Autodesk Inventor part; units mm, degrees
ref_plane "C3_XY" through (39.5, 0, 0) normal (-1, 0, 0) x (0, 0, -1)
ref_plane "C3_YZ" through (39.5, 0, 0) normal (0, 0, -1) x (0, -1, 0)
ref_plane "C3_ZX" through (39.5, 0, 0) normal (0, -1, 0) x (-1, 0, 0)
sketch "Sketch_1" plane through (0, 0, 0) normal (0, 0, 1) x (1, 0, 0)
  line L0 (39.5, 0) -> (0, 0)
  line L1 (0, 0) -> (0, 3)
  line L2 (0, 3) -> (0.5485, 3.95)
  line L3 (0.5485, 3.95) -> (38.9515, 3.95)
  line L4 (38.9515, 3.95) -> (39.5, 3)
  line L5 (39.5, 3) -> (39.5, 0)
  line L6 (39.5, 0) -> (0, 0)
revolve "Revolution1" add sketch "Sketch_1" angle 360 about axis through (39.5, 0, 0) along (1, 0, 0)
sketch "Sketch_2" plane through (0, 0, 0) normal (1, 0, 0) x (0, 1, 0)
  line L0 (6, 6) -> (-6, 6)
  line L1 (-6, 6) -> (-6, -6)
  line L2 (-6, -6) -> (6, -6)
  line L3 (6, -6) -> (6, 6)
  line L4 (-1.7321, 3) -> (-3.4641, 0)
  line L5 (-3.4641, 0) -> (-1.7321, -3)
  line L6 (-1.7321, -3) -> (1.7321, -3)
  line L7 (1.7321, -3) -> (3.4641, 0)
  line L8 (3.4641, 0) -> (1.7321, 3)
  line L9 (1.7321, 3) -> (-1.7321, 3)
extrude "Extrusion1" cut sketch "Sketch_2" along normal blind 39.5
sketch "Sketch3" plane through (0, 0, 0) normal (-1, 0, 0) x (0, 0, 1)
  point P0 (0, 0)
hole "Hole1" at (0, 0, 0) direction (1, 0, 0) diameter 2.459 depth 8.2901 tip angle 120 countersink diameter 3 countersink angle 90
sketch "Sketch4" plane through (39.5, 0, 0) normal (1, 0, 0) x (0, 0, -1)
  point P0 (0, 0)
hole "Hole2" at (39.5, 0, 0) direction (-1, 0, 0) diameter 2.459 depth 8.2901 tip angle 120 countersink diameter 3 countersink angle 90
ref_plane "C3_XY" through (39.5, 0, 0) normal (-1, 0, 0) x (0, 0, -1)
ref_plane "C3_YZ" through (39.5, 0, 0) normal (0, 0, -1) x (0, -1, 0)
ref_plane "C3_ZX" through (39.5, 0, 0) normal (0, -1, 0) x (-1, 0, 0)
properties part number "SLSBF6-39.5-M3-N3"
Input: part model. Units: mm. Frame: model coordinates. A direction names the side the tool comes from. Give positions to 0.01 mm unless a question says otherwise; leave off trailing zeros. Order: outer loops, then holes, each group sorted by start corner. A loop starts at its lowest first (then second) coordinate and runs counter-clockwise, first axis right, second up. Notation, with made-up numbers: M -35,28.5 L -11,28.5 A35 ccw -11,62.5 Z; hole C 21,55.5 d1. An arc over 180 degrees is marked long. Return JSON: item names as keys, results as strings.
1) Line query: L1, parallel to Z at x = 5.5, y = 0; L2, parallel to Z at x = 32, y = 0.5; L3, parallel to Y at x = 3.5, z = -0.8. Output: solid intervals per line, ascending. Write a range as [from, to].
Taken from the geometry:
{"L1": "z = [-3, -1.23], [1.23, 3]", "L2": "z = [-3, -1.12], [1.12, 3]", "L3": "y = [-3, -0.93], [0.93, 3]"}
2) Access query for faces 1 (the face through (0.076, 3.131, -0.069)), 2 (the face through (35.164, 0.748, 0.976)). Directions: +Z, -Z, +X, -X, +Y, -Y. A direction counts if a zero-diameter tool reaches every point of the face in a straight line with its end or side. Return the directions, or none.
Taken from the geometry:
{"face 1": "-X, +Y", "face 2": "+X"}
3) Mould query, pull axis Y, two halves, no side actions, for faces 3 (the face through (4.336, 0.748, -0.976)), 4 (the face through (19.5, 2.6, 1.5)), 5 (the face through (19.5, -2.6, 1.5)). Classes: released by +Y, released by -Y, zero draft, split by the parting line, or undercut.
Taken from the geometry:
{"face 3": "undercut", "face 4": "released by +Y", "face 5": "released by -Y"}
4) Section query B-B on x = 9.5. Output: boundary loops of the cut face in (y, z), and give its area (3 significant figures).
Taken from the geometry:
{"outline": "M -3.46,0 L -1.73,-3 L 1.73,-3 L 3.46,0 L 1.73,3 L -1.73,3 Z", "area": "31.2 mm2"}
5) Section query A-A on x = 37.5. Output: boundary loops of the cut face in (y, z), and give its area (3 significant figures).
Taken from the geometry:
{"outline": "M -3.46,0 L -1.73,-3 L 1.73,-3 L 3.46,0 L 1.73,3 L -1.73,3 Z; hole C 0,0 d2.46", "area": "26.4 mm2"}
6) Contact query for flat-ended pins moving along their axis: pin 1 (2 mm diameter, centred on x = 27.5, z = -1.5, fed in from -Y); pin 2 (2 mm diameter, centred on y = 0, z = 0, fed in from +X); pin 3 (3 mm diameter, centred on x = 18.5, y = -2, fed in from +Z); pin 4 (3 mm diameter, centred on x = 16.5, z = 2, fed in from +Y). Output: stop coordinate, or through.
Taken from the geometry:
{"pin 1": "stops at y = -3.18", "pin 2": "stops at x = 31.08", "pin 3": "stops at z = 3", "pin 4": "stops at y = 3.18"}
